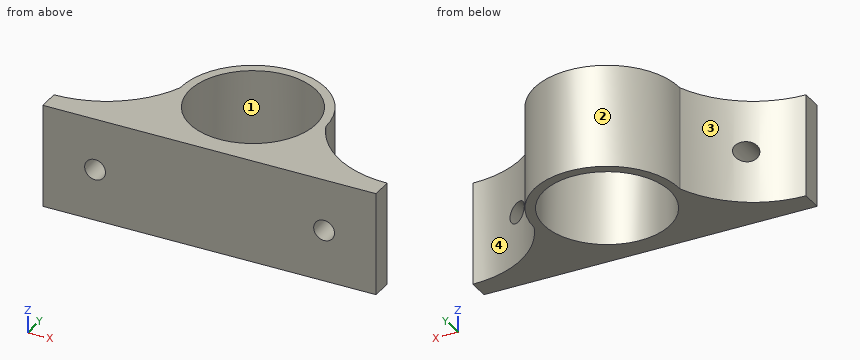
```python
from build123d import *

# Parameters (mm, degrees)
F0_R     = 15.25
F1_DEPTH = 25
F2_R     = 2.5
F3_DEPTH = 25


with BuildPart() as f1:
    # F0 (on Top) → F1 (new body)
    with BuildSketch(Plane.XY):
        with BuildLine():
            ThreePointArc((40, -15), (26.479183, -10.906226), (17.5, 0))
            ThreePointArc((17.5, 0), (0, 17.5), (-17.5, 0))
            ThreePointArc((-17.5, 0), (-26.479183, -10.906226), (-40, -15))
            Line((-40, -15), (-40, -20))
            Line((-40, -20), (40, -20))
            Line((40, -20), (40, -15))
        make_face()
        Circle(F0_R, mode=Mode.SUBTRACT)
    extrude(amount=F1_DEPTH)

    # F2 (on Front) → F3 (cut)
    with BuildSketch(Plane.XZ):
        with Locations((27.5, 12.5)):
            Circle(F2_R)
        with Locations((-27.5, 12.5)):
            Circle(F2_R)
    extrude(amount=F3_DEPTH, mode=Mode.SUBTRACT)


solid = f1.part
```
Part model, mm, in its own coordinate system. Face numbers are marked on the shaded views. Round coordinates to 2 decimals unless told otherwise and drop trailing zeros. Order: outer loops, then holes, each group sorted by start corner. A loop starts at its lowest first (then second) coordinate and runs counter-clockwise, first axis right, second up. Notation, with made-up numbers: M -19,-24 L 14,-24 A8 cw 14,-19 Z; hole C -12.5,-9.75 d1. An arc over 180 degrees is marked long. Answer in a Markdown table with one row per item. Add a question column.
Q1. Cut at A-A on z = 20.75. Give the cut face in (x, y) (3 decimals), and give its area (3 significant figures).
Q2. Cut at C-C on y = -5. Give the cut face in (x, z).
Q3. Wall check: L1, parallel to X at y = -16.5, z = 12.5; L2, parallel to Y at x = 0, z = 16.5; L3, parallel to X at y = -2, z = 20. Give the ranges that are in metal, low to high. Write a range as from..to.
Q4. Mould opens along X. For the marked faces 1, 2, 3 and 4 say: +X half, -X half, draft (parallel to the pull), parting line (faces both ways), or undercut.
Q5. Pin check, flat tip, straight feed: pin 1 (1 mm diameter, centred on y = 7, z = 19.5, fed in from -X). Stop position of the tip, or through.
Q6. Cut at B-B on x = 0. Give the cut face in (y, z).
Q7. Cut at D-D on z = 12.5. Give the cut face in (x, y) (3 decimals), and give its area (3 significant figures).
Established:
| question | item | result |
|---|---|---|
| 1 | outline | M -40,-20 L 40,-20 L 40,-15 A24.375 cw 17.5,0 A17.5 ccw -17.5,0 A24.375 cw -40,-15 Z; hole C 0,0 d30.5 |
| 1 | area | 863 mm2 |
| 2 | outline | M -20.31,0 L -14.41,0 L -14.41,25 L -20.31,25 Z; M 14.41,0 L 20.31,0 L 20.31,25 L 14.41,25 Z |
| 3 | L1 | x = -40..-30, -25..25, 30..40 |
| 3 | L2 | y = -20..-15.25, 15.25..17.5 |
| 3 | L3 | x = -18.44..-15.12, 15.12..18.44 |
| 4 | face 1 | undercut |
| 4 | face 2 | parting line |
| 4 | face 3 | -X half |
| 4 | face 4 | +X half |
| 5 | pin 1 | stops at x = -16.25 |
| 6 | outline | M -20,0 L -15.25,0 L -15.25,25 L -20,25 Z; M 15.25,0 L 17.5,0 L 17.5,25 L 15.25,25 Z |
| 7 | outline | M -40,-20 L -30,-20 L -30,-12.854 A24.375 cw -40,-15 Z; M -25,-20 L 25,-20 L 25,-9.838 A24.375 cw 17.5,0 A17.5 ccw -17.5,0 A24.375 cw -25,-9.838 Z; M 30,-20 L 40,-20 L 40,-15 A24.375 cw 30,-12.854 Z; hole C 0,0 d30.5 |
| 7 | area | 777 mm2 |
